from build123d import *

# Parameters (mm, degrees)
F0_R     = 11.025
F1_DEPTH = 7


with BuildPart() as f1:
    # F0 (on Top) → F1 (new body)
    with BuildSketch(Plane.XY):
        with BuildLine():
            ThreePointArc((12.8607921453, -2.061710365), (12.9838831161, -1.0341196545), (13.0249999706, 0))
            ThreePointArc((13.0249999706, 0), (6.5569336334, 11.254210126), (-6.423329526, 11.330995633))
            Line((-6.423329526, 11.330995633), (-12.3569446603, 4.1178323055))
            ThreePointArc((-12.3569446603, 4.1178323055), (-8.0930947102, -10.2055103863), (6.8250050843, -11.0936887388))
            Line((6.8250050843, -11.0936887388), (6.8250050843, -10.7323580555))
            Line((6.8250050843, -10.7323580555), (12.8607921453, -2.061710365))
        make_face()
        Circle(F0_R, mode=Mode.SUBTRACT)
        with BuildLine():
            Line((-12.3569446603, 4.1178323055), (-6.423329526, 11.330995633))
            ThreePointArc((-6.423329526, 11.330995633), (-10.0589316493, 8.2745705815), (-12.3569446603, 4.1178323055))
        make_face()
        with BuildLine():
            ThreePointArc((-12.3569446603, 4.1178323055), (-10.0589316493, 8.2745705815), (-6.423329526, 11.330995633))
            Line((-6.423329526, 11.330995633), (-6.1813540831, 11.6251516156))
            Line((-6.1813540831, 11.6251516156), (-6.1813540831, 23.2478915714))
            Line((-6.1813540831, 23.2478915714), (-14.1813540831, 27.6478952728))
            Line((-14.1813540831, 27.6478952728), (-6.1813540831, 27.6478952728))
            Line((-6.1813540831, 27.6478952728), (-6.1813540831, 39.2706352286))
            Line((-6.1813540831, 39.2706352286), (-14.1813540831, 50.762952771))
            Line((-14.1813540831, 50.762952771), (-22.1813540831, 39.2706352286))
            Line((-22.1813540831, 39.2706352286), (-22.1813540831, 27.6478952728))
            Line((-22.1813540831, 27.6478952728), (-14.1813540831, 23.2478915714))
            Line((-14.1813540831, 23.2478915714), (-22.1813540831, 23.2478915714))
            Line((-22.1813540831, 23.2478915714), (-22.1813540831, 11.6251516156))
            Line((-22.1813540831, 11.6251516156), (-14.1813540831, 1.900000032))
            Line((-14.1813540831, 1.900000032), (-12.3569446603, 4.1178323055))
        make_face()
        Polygon((-14.5165706053, 22.92711474), (-14.1813540831, 22.92711474), (-13.8461375609, 22.92711474), (-13.8461375609, 11.9459284469), (-14.1813540831, 11.9459284469), (-14.5165706053, 11.9459284469), align=None, mode=Mode.SUBTRACT)
        Polygon((-13.8690257445, 28.0980104581), (-14.1813540831, 28.0980104581), (-14.4936824217, 28.0980104581), (-14.4936824217, 38.8205200434), (-14.1813540831, 38.8205200434), (-13.8690257445, 38.8205200434), align=None, mode=Mode.SUBTRACT)
        with BuildLine():
            Line((14.8250050843, 0.759959487), (12.8607921453, -2.061710365))
            ThreePointArc((12.8607921453, -2.061710365), (10.829441882, -7.2369753873), (6.8250050843, -11.0936887388))
            Line((6.8250050843, -11.0936887388), (6.8250050843, -22.3550980112))
            Line((6.8250050843, -22.3550980112), (14.8250050843, -26.7551017127))
            Line((14.8250050843, -26.7551017127), (6.8250050843, -26.7551017127))
            Line((6.8250050843, -26.7551017127), (6.8250050843, -38.3778416685))
            Line((6.8250050843, -38.3778416685), (14.8250050843, -48.102993252))
            Line((14.8250050843, -48.102993252), (22.8250050843, -38.3778416685))
            Line((22.8250050843, -38.3778416685), (22.8250050843, -26.7551017127))
            Line((22.8250050843, -26.7551017127), (14.8250050843, -22.3550980112))
            Line((14.8250050843, -22.3550980112), (22.8250050843, -22.3550980112))
            Line((22.8250050843, -22.3550980112), (22.8250050843, -10.7323580555))
            Line((22.8250050843, -10.7323580555), (14.8250050843, 0.759959487))
        make_face()
        with BuildLine():
            ThreePointArc((6.8250050843, -11.0936887388), (10.829441882, -7.2369753873), (12.8607921453, -2.061710365))
            Line((12.8607921453, -2.061710365), (6.8250050843, -10.7323580555))
            Line((6.8250050843, -10.7323580555), (6.8250050843, -11.0936887388))
        make_face()
    extrude(amount=F1_DEPTH)


solid = f1.part
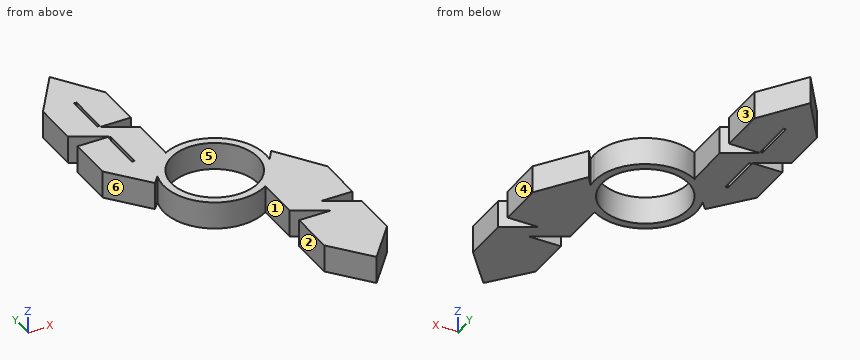
For this review, take the finished solid that the model builds, in its own axes (mm). Face numbers are marked on the shaded views. A direction names the side the tool comes from. Give positions to 0.01 mm unless a question says otherwise; leave off trailing zeros. Order: outer loops, then holes, each group sorted by start corner. A loop starts at its lowest first (then second) coordinate and runs counter-clockwise, first axis right, second up. Notation, with made-up numbers: (33.5, -17.5) - (79.5, -17.5) arc R26 ccw to (79.5, 0.5) - close; hole circle Ø10 at (-15.5, 39.5). An arc over 180 degrees is marked (long way). Answer as a JSON object with one key per item and string values. Group by question number.
Item 1: Draft analysis for pull direction Y (two halves, no side actions). For the marked faces 4, 5 and 6, state which applies: pulls with the +Y half, pulls with the -Y half, needs draft (parallel to the pull), parting line crosses it, or undercut.
Item 2: Machinability: for the marked faces 1, 2 and 3, which of the approach directions +Z, -Z, +X, -X, +Y, -Y give a long, thin tool a straight path to every point of the face, cutting with its end or side? Answer none if there is none.
Item 3: Wall thickness on line 1 along Y through (x, z) = (0, 5.25) (3 decimals); line 2 along Y through (x, z) = (8.5, 6.5); line 3 along X through (y, z) = (-36.5, 1.25) (3 decimals): over which ranges is each line inside the solid? List them lowest first.
Item 4: Take a section at C-C on x = -18. Give the boundary of the cut face in (y, z), and give its area (3 significant figures).
Item 5: Take a section at B-B on z = 5.5. Give the number of separate pieces and of enclosed holes in the cut face, and give its area (3 significant figures).
Item 6: Take a section at A-A on x = 0. Give the boundary of the cut face in (y, z) (3 decimals), and give its area (3 significant figures).
Item 7: Take a section at D-D on y = 40.5. Give the boundary of the cut face in (x, z), and give its area (3 significant figures).
Item 8: Clearance check with flat-ended pins moving along their axes: pin 1 Ø1.5 at (y, z) = (12, 3) entering from +X; pin 2 Ø1.5 at (x, z) = (-4.5, 5) entering from +Y; pin 3 Ø3.5 at (y, z) = (-15, 5) entering from -X (3 decimals). State where each tip first meets the part, or that it passes through.
Reported:
{
 "1": {"face 4": "needs draft", "face 5": "undercut", "face 6": "pulls with the -Y half"},
 "2": {"face 1": "+Z, -Z, -Y", "face 2": "+Z, -Z, -X, -Y", "face 3": "+Z, -Z, +X, +Y"},
 "3": {"line 1": "-13.025 to -11.025, 11.025 to 13.025", "line 2": "-40.41 to -26.76, -23.28 to -7.02, 7.02 to 9.87", "line 3": "6.825 to 22.825"},
 "4": {"outline": "(6.54, 0) - (23.25, 0) - (23.25, 7) - (6.54, 7) - close; (25.35, 0) - (45.28, 0) - (45.28, 7) - (25.35, 7) - close", "area": "256 mm^2"},
 "5": {"separate pieces": "1", "enclosed holes": "3", "area": "1,280 mm^2"},
 "6": {"outline": "(-13.025, 0) - (-11.025, 0) - (-11.025, 7) - (-13.025, 7) - close; (11.025, 0) - (13.025, 0) - (13.025, 7) - (11.025, 7) - close", "area": "28.0 mm^2"},
 "7": {"outline": "(-21.33, 0) - (-7.04, 0) - (-7.04, 7) - (-21.33, 7) - close", "area": "100 mm^2"},
 "8": {"pin 1": "x = 6.56", "pin 2": "y = 12.47", "pin 3": "x = 6.825"}
}
